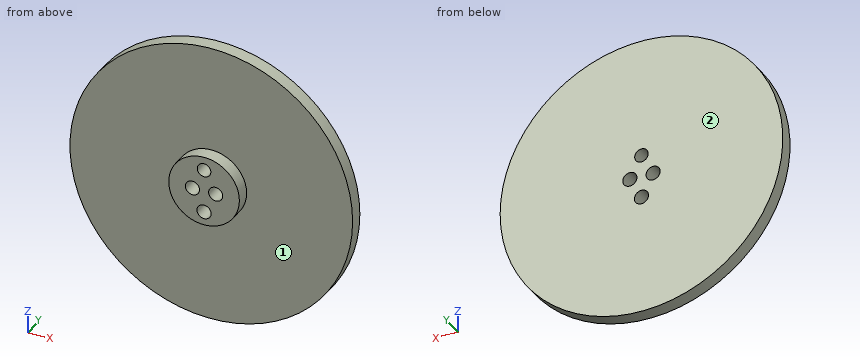
```python
from build123d import *

# Parameters (mm, degrees)
SKETCH1_R           = 15.875
BOSS_EXTRUDE1_DEPTH = 6.35
SKETCH2_R           = 63.5
BOSS_EXTRUDE2_DEPTH = 6.35
SKETCH9_R           = 3.048
CUT_EXTRUDE1_DEPTH  = 13.7
SKETCH10_R          = 3.175
CUT_EXTRUDE2_DEPTH  = 12.7
SKETCH11_R          = 3.175
CUT_EXTRUDE3_DEPTH  = 12.7
SKETCH12_R          = 3.175
CUT_EXTRUDE4_DEPTH  = 12.7


with BuildPart() as part:
    # Sketch1 → Boss-Extrude1 (new body)
    with BuildSketch(Plane(origin=(0, 0, 0), x_dir=(1, 0, 0), z_dir=(0, 1, 0))):
        Circle(SKETCH1_R)
    extrude(amount=BOSS_EXTRUDE1_DEPTH)

    # Sketch2 → Boss-Extrude2 (add)
    with BuildSketch(Plane(origin=(0, 6.35, 0), x_dir=(1, 0, 0), z_dir=(0, 1, 0))):
        Circle(SKETCH2_R)
    extrude(amount=BOSS_EXTRUDE2_DEPTH)

    # Sketch9 → Cut-Extrude1 (cut, through all)
    with BuildSketch(Plane.XZ):
        with Locations((0, 9.779)):
            Circle(SKETCH9_R)
    extrude(amount=-CUT_EXTRUDE1_DEPTH, mode=Mode.SUBTRACT)

    # Sketch10 → Cut-Extrude2 (cut)
    with BuildSketch(Plane.XZ):
        with Locations((0, -9.779)):
            Circle(SKETCH10_R)
    extrude(amount=-CUT_EXTRUDE2_DEPTH, mode=Mode.SUBTRACT)

    # Sketch11 → Cut-Extrude3 (cut)
    with BuildSketch(Plane.XZ):
        with Locations((-5.22478, 0)):
            Circle(SKETCH11_R)
    extrude(amount=-CUT_EXTRUDE3_DEPTH, mode=Mode.SUBTRACT)

    # Sketch12 → Cut-Extrude4 (cut)
    with BuildSketch(Plane.XZ):
        with Locations((5.22478, 0)):
            Circle(SKETCH12_R)
    extrude(amount=-CUT_EXTRUDE4_DEPTH, mode=Mode.SUBTRACT)


solid = part.part
```
Source: CAD feature listing. Evaluate the final solid. Frame: model axes, mm. Face numbers are marked on the shaded views. A direction names the side the tool comes from. Round coordinates to 2 decimals unless told otherwise and drop trailing zeros. Loops run counter-clockwise (first coordinate to the right, second up) from the corner with the lowest first, then second, coordinate; pieces in that order, holes last.
1. Section query C-C on y = 3.5. Output: boundary loops of the cut face in (x, z) (3 decimals), and give its area (3 significant figures).
2. Section query D-D on x = -25. Output: boundary loops of the cut face in (y, z).
3. Ray query, L1, parallel to X at y = 10, z = -1; L2, parallel to Z at x = 2.5, y = 8.25; L3, parallel to Z at x = 1.5, y = 9.25. Return the intervals inside material, ascending.
4. Section query B-B on z = 0. Output: boundary loops of the cut face in (x, y) (3 decimals).
5. Contact query for flat-ended pins moving along their axis: pin 1 (1.5 mm diameter, centred on y = 8.5, z = 26.5, fed in from -X); pin 2 (3 mm diameter, centred on x = -10, y = 7.5, fed in from -Z); pin 3 (4 mm diameter, centred on y = 4.5, z = 2.5, fed in from -X). Output: stop coordinate, or through.
6. Access query for the marked faces 1 and 2. Directions: +Z, -Z, +X, -X, +Y, -Y. A direction counts if a zero-diameter tool reaches every point of the face in a straight line with its end or side. Return the directions, or none.
7. Section query A-A on x = 0. Output: boundary loops of the cut face in (y, z) (3 decimals).
Answers below:
1. outline: circle Ø31.75 at (0, 0); hole circle Ø6.35 at (-5.225, 0); hole circle Ø6.35 at (0, -9.779); hole circle Ø6.096 at (0, 9.779); hole circle Ø6.35 at (5.225, 0)
1. area: 668 mm2
2. outline: (6.35, -58.37) - (12.7, -58.37) - (12.7, 58.37) - (6.35, 58.37) - close
3. L1: x = -63.49 to -8.24, -2.21 to 2.21, 8.24 to 63.49
3. L2: z = -63.45 to -11.74, -7.82 to -1.63, 1.63 to 8.04, 11.52 to 63.45
3. L3: z = -63.48 to -12.58, -6.98 to 7.13, 12.43 to 63.48
4. outline: (-63.5, 6.35) - (-15.875, 6.35) - (-15.875, 0) - (-8.4, 0) - (-8.4, 12.7) - (-63.5, 12.7) - close; (-2.05, 0) - (2.05, 0) - (2.05, 12.7) - (-2.05, 12.7) - close; (8.4, 0) - (15.875, 0) - (15.875, 6.35) - (63.5, 6.35) - (63.5, 12.7) - (8.4, 12.7) - close
5. pin 1: stops at x = -58.04
5. pin 2: stops at z = -62.93
5. pin 3: stops at x = -63.48
6. face 1: -Y
6. face 2: +Z, -Z, +X, -X, +Y
7. outline: (0, -15.875) - (6.35, -15.875) - (6.35, -63.5) - (12.7, -63.5) - (12.7, -12.954) - (0, -12.954) - close; (0, -6.604) - (12.7, -6.604) - (12.7, 6.731) - (0, 6.731) - close; (0, 12.827) - (12.7, 12.827) - (12.7, 63.5) - (6.35, 63.5) - (6.35, 15.875) - (0, 15.875) - close
